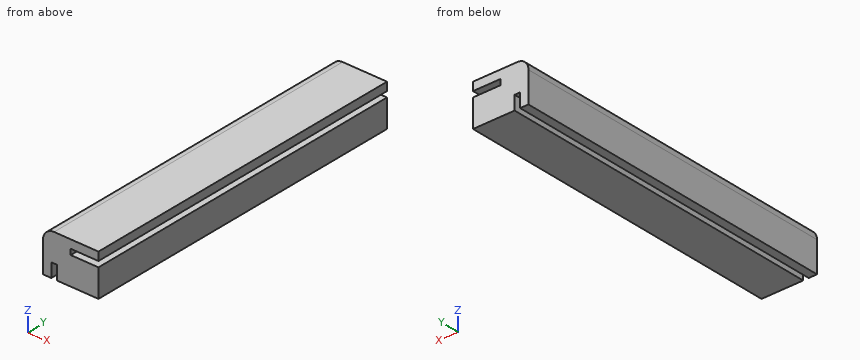
```python
from build123d import *

# Parameters (mm, degrees)
F0_W     = 25.4
F0_H     = 152.4
F1_DEPTH = 19.05
F2_W     = 12.7
F2_H     = 2.54
F2_W_2   = 2.54
F2_H_2   = 6.35
F3_DEPTH = 177.8
F4_R     = 5.08


with BuildPart() as f1:
    # F0 (on Top) → F1 (new body)
    with BuildSketch(Plane.XY):
        Rectangle(F0_W, F0_H)
    extrude(amount=F1_DEPTH)

    # F2 (on face) → F3 (cut)
    with BuildSketch(Plane.XZ.offset(76.2)):
        with Locations((6.35, 13.97)):
            Rectangle(F2_W, F2_H)
        with Locations((-7.62, 3.175)):
            Rectangle(F2_W_2, F2_H_2)
    extrude(amount=-F3_DEPTH, mode=Mode.SUBTRACT)

    # F4
    f4_edges = [f1.edges().sort_by_distance(p)[0] for p in [
        (-12.7, 0, 19.05),
    ]]
    fillet(f4_edges, radius=F4_R)


solid = f1.part
```
Source: CAD feature listing. Evaluate the final solid. Frame: model axes, mm. Give positions to 0.01 mm unless a question says otherwise; leave off trailing zeros. Write each loop counter-clockwise with the first axis right and the second up, starting at its lowest first coordinate (ties: lowest second). Pieces come first, ordered by that corner, then holes.
1. Section query C-C (y = -17). Return the cut outline in (x, z), then the cut area to 3 significant figures.
2. Section query A-A (x = 8.75). Return the cut outline in (y, z), then the cut area to 3 significant figures.
3. First-contact query: pin 1 (0.8 mm diameter, centred on y = 36.5, z = 14, fed in from +X). Flat tip, straight axial feed; report the tip coordinate or a pass-through.
4. Material intervals for line 1 along X through (y, z) = (7.5, 1); line 2 along Z through (x, y) = (2, 4), sorted ascending.
5. Section query D-D (z = 17.25). Return the cut outline in (x, y), then the cut area to 3 significant figures.
6. Section query B-B (z = 2.75). Return the cut outline in (x, y).
Output values:
1. outline: (-12.7, 0) - (-8.89, 0) - (-8.89, 6.35) - (-6.35, 6.35) - (-6.35, 0) - (12.7, 0) - (12.7, 12.7) - (0, 12.7) - (0, 15.24) - (12.7, 15.24) - (12.7, 19.05) - (-7.62, 19.05) arc R5.08 ccw to (-12.7, 13.97) - close
1. area: 430 mm2
2. outline: (-76.2, 0) - (76.2, 0) - (76.2, 12.7) - (-76.2, 12.7) - close; (-76.2, 15.24) - (76.2, 15.24) - (76.2, 19.05) - (-76.2, 19.05) - close
2. area: 2,520 mm2
3. pin 1: stops at x = 0
4. line 1: x = -12.7 to -8.89, -6.35 to 12.7
4. line 2: z = 0 to 12.7, 15.24 to 19.05
5. outline: (-11.5, -76.2) - (12.7, -76.2) - (12.7, 76.2) - (-11.5, 76.2) - close
5. area: 3,690 mm2
6. outline: (-12.7, -76.2) - (-8.89, -76.2) - (-8.89, 76.2) - (-12.7, 76.2) - close; (-6.35, -76.2) - (12.7, -76.2) - (12.7, 76.2) - (-6.35, 76.2) - close
